```python
from build123d import *

# Parameters (mm, degrees)
SKETCH_1_R      = 7.744401216
EXTRUDE_1_DEPTH = 10
FILLET_1_R      = 10


with BuildPart() as part:
    # 草图1 → 凸台-拉伸1 (new body)
    with BuildSketch(Plane(origin=(0, 0, 0), x_dir=(1, 0, 0), z_dir=(0, 1, 0))):
        with BuildLine():
            ThreePointArc((14.606255334, 10), (-17.701488493, 0), (14.606255334, -10))
            Line((14.606255334, -10), (130.028894825, -10))
            ThreePointArc((130.028894825, -10), (162.336638652, 0), (130.028894825, 10))
            Line((130.028894825, 10), (14.606255334, 10))
        make_face()
        with Locations(Location((0, 0, 0), (0, 0, 270))):
            Circle(SKETCH_1_R, mode=Mode.SUBTRACT)
        with Locations(Location((144.635150159, 0, 0), (0, 0, 270))):
            Circle(SKETCH_1_R, mode=Mode.SUBTRACT)
    extrude(amount=EXTRUDE_1_DEPTH)

    # 圆角1
    fillet_1_edges = [part.edges().sort_by_distance(p)[0] for p in [
        (130.028894825, 5, -10),
        (130.028894825, 5, 10),
        (14.606255334, 5, 10),
        (14.606255334, 5, -10),
    ]]
    fillet(fillet_1_edges, radius=FILLET_1_R)


solid = part.part
```
Part model, mm, in its own coordinate system. A direction names the side the tool comes from. Round coordinates to 2 decimals unless told otherwise and drop trailing zeros. Loops run counter-clockwise (first coordinate to the right, second up) from the corner with the lowest first, then second, coordinate; pieces in that order, holes last.
1. 3-axis set-ups, long thin cutter, end or side, ignore diameter. For faces 1 (the face through (71, 10, 0)), 2 (the face through (73, 5, -10)), 3 (the face through (129.147, 5.07, 10.701)): which of +Z, -Z, +X, -X, +Y, -Y reach the whole face in a straight line?
Solutions:
face 1: +Z, -Z, +X, -X, +Y
face 2: -Z, +Y, -Y
face 3: +Z, +Y, -Y
2. Slice it at A-A (x = 0). Give the cut face in (y, z), and give its area (3 significant figures).
Solutions:
outline: (0, -17.7) - (10, -17.7) - (10, -7.74) - (0, -7.74) - close; (0, 7.74) - (10, 7.74) - (10, 17.7) - (0, 17.7) - close
area: 199 mm2
3. Slice it at B-B (z = 0). Give the cut face in (x, y), and give its area (3 significant figures).
Solutions:
outline: (-17.7, 0) - (-7.74, 0) - (-7.74, 10) - (-17.7, 10) - close; (7.74, 0) - (136.89, 0) - (136.89, 10) - (7.74, 10) - close; (152.38, 0) - (162.34, 0) - (162.34, 10) - (152.38, 10) - close
area: 1,490 mm2
4. Two-plate mould, pull along Z, no slides. Class faces 4 (the face through (72, 5, 10)), 5 (the face through (7.68, 4.93, -1.01)), 6 (the face through (129.147, 5.07, -10.701)): pulls with the +Z half, pulls with the -Z half, needs draft (parallel to the pull), parting line crosses it, or undercut.
Solutions:
face 4: pulls with the +Z half
face 5: undercut
face 6: pulls with the -Z half
5. Slice it at C-C (y = 7). Give the cut face in (x, z), and give its area (3 significant figures).
Solutions:
outline: (12.25, -12.78) arc R10 cw to (19.17, -10) - (125.47, -10) arc R10 cw to (132.39, -12.78) arc R17.7 ccw (long way) to (132.39, 12.78) arc R10 cw to (125.47, 10) - (19.17, 10) arc R10 cw to (12.25, 12.78) arc R17.7 ccw (long way) to start; hole circle Ø15.49 at (0, 0); hole circle Ø15.49 at (144.64, 0)
area: 3,830 mm2
6. Slice it at D-D (x = 79). Give the cut face in (y, z), and give its area (3 significant figures).
Solutions:
outline: (0, -10) - (10, -10) - (10, 10) - (0, 10) - close
area: 200 mm2
7. Drill centre lines: line 1 along X through (y, z) = (1, -1.5); line 2 along X through (y, z) = (8.75, -7); line 3 along Z through (x, y) = (77, 5.5). Where is each one in solid material? Low to high.
Solutions:
line 1: x = -17.64 to -7.6, 7.6 to 137.04, 152.23 to 162.27
line 2: x = -16.26 to -3.31, 3.31 to 141.32, 147.95 to 160.89
line 3: z = -10 to 10
